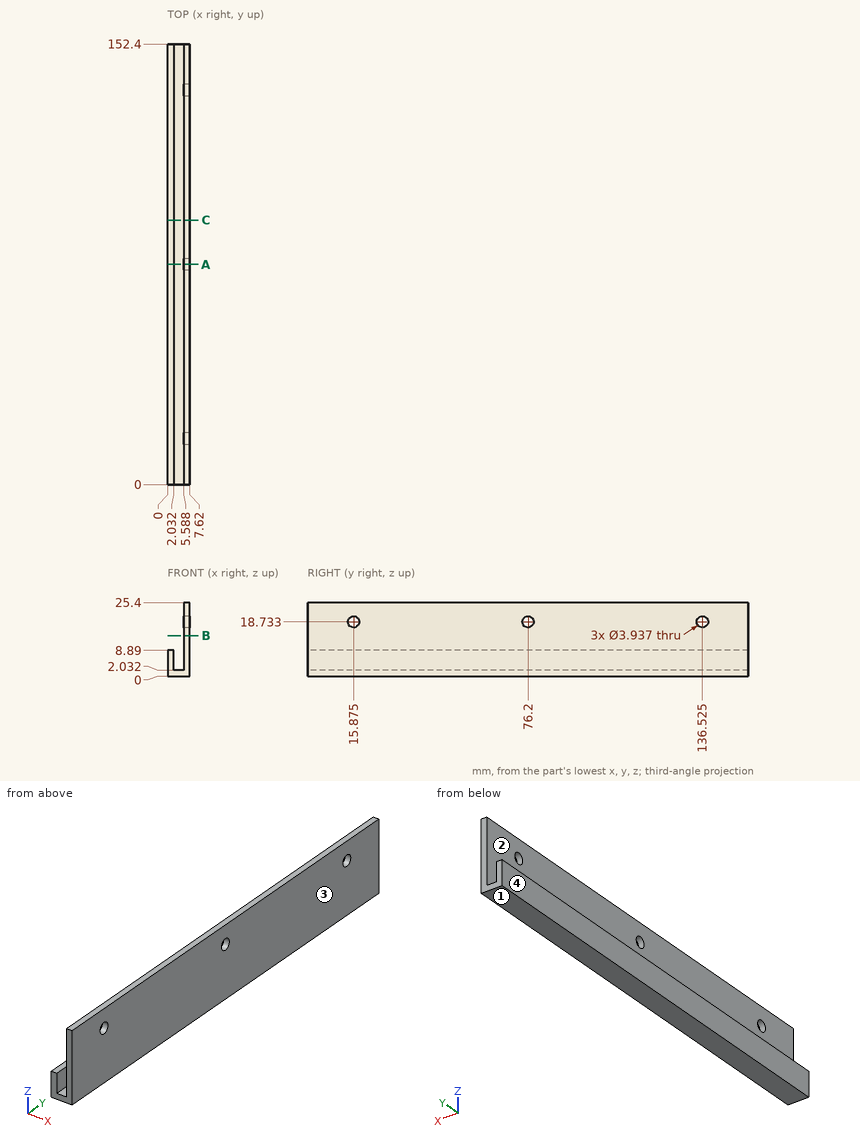
Print and shaded views of the part. All mm, measured from the part's lowest x, y and z. Round coordinates to 2 decimals unless told otherwise and drop trailing zeros. Write each loop counter-clockwise with the first axis right and the second up, starting at its lowest first coordinate (ties: lowest second). Pieces come first, ordered by that corner, then holes. Notation, with made-up numbers: M 74,-0.5 L 104,-0.5 A16 ccw 104,16.5 Z; hole C 66,-30 d4. An arc over 180 degrees is marked long. Use a Markdown table: item, result. Add a question column.
1. Slice it at A-A on y = 76.2. Give the cut face in (x, z) (1 decimal).
2. Drill centre lines: probe 1 along Z at (x, y) = (6.4, 76.2) (1 decimal); probe 2 along X at (y, z) = (100, 5.5); probe 3 along X at (y, z) = (30.5, 23.5). Where is each one in solid material? Low to high.
3. Slice it at C-C on y = 91.5. Give the cut face in (x, z).
4. Pull direction X, two halves, no side cores. Call the marked faces 1, 2, 3 and 4: released by +X, released by -X, zero draft, split by the parting line, or undercut.
5. Slice it at B-B on z = 14. Give the cut face in (x, y).
6. Flat gauge pins, fed straight in: P1, Ø4, axis at x = 3, z = 18, coming from the -Y side; P2, Ø1.6, axis at x = 0.5, y = 59, coming from the +Z side. Where does each tip first touch, or does it go through?
Reply:
| question | item | result |
|---|---|---|
| 1 | outline | M 0,0 L 7.6,0 L 7.6,16.8 L 5.6,16.8 L 5.6,2 L 2,2 L 2,8.9 L 0,8.9 Z; M 5.6,20.7 L 7.6,20.7 L 7.6,25.4 L 5.6,25.4 Z |
| 2 | probe 1 | z = 0 to 16.8, 20.7 to 25.4 |
| 2 | probe 2 | x = 0 to 2.03, 5.59 to 7.62 |
| 2 | probe 3 | x = 5.59 to 7.62 |
| 3 | outline | M 0,0 L 7.62,0 L 7.62,25.4 L 5.59,25.4 L 5.59,2.03 L 2.03,2.03 L 2.03,8.89 L 0,8.89 Z |
| 4 | face 1 | zero draft |
| 4 | face 2 | undercut |
| 4 | face 3 | released by +X |
| 4 | face 4 | released by -X |
| 5 | outline | M 5.59,0 L 7.62,0 L 7.62,152.4 L 5.59,152.4 Z |
| 6 | P1 | passes through |
| 6 | P2 | stops at z = 8.89 |
